Can you work these out from the model? Positions are in its coordinate system, mm. Face numbers are marked on the shaded views. A direction names the side the tool comes from. Give positions to 0.01 mm unless a question says otherwise; leave off trailing zeros. Write each loop counter-clockwise with the first axis right and the second up, starting at its lowest first coordinate (ties: lowest second). Pieces come first, ordered by that corner, then holes. Notation, with made-up numbers: (5.25, 37) -> (42.25, 37) arc R27 cw to (42.25, 64) -> close; hole circle Ø4 at (89, -1). An arc over 180 degrees is marked (long way). One line per item, written item: value.
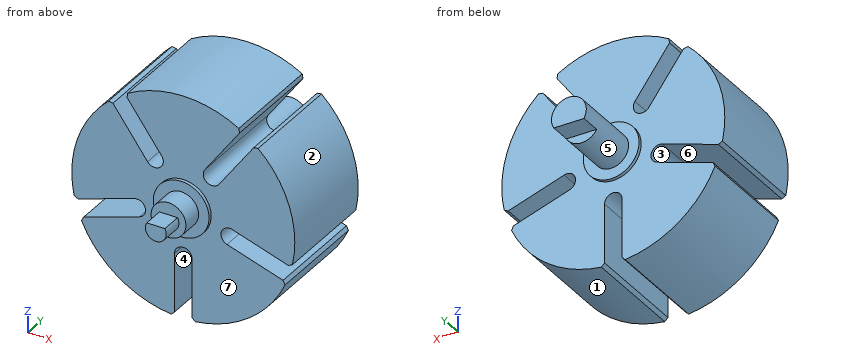
from build123d import *

# Parameters (mm, degrees)
SKETCH_1_R               = 16
EXTRUDE_1_DEPTH          = 15
SKETCH_2_R               = 4
EXTRUDE_2_DEPTH          = 0.5
EXTRUDE_START            = 0.5
SKETCH_3_R               = 4
EXTRUDE_3_DEPTH          = 0.5
SKETCH_4_R               = 2.5
EXTRUDE_4_DEPTH          = 10
EXTRUDE_START_2          = 3
SKETCH_5_R               = 2.5
EXTRUDE_5_DEPTH          = 3
CUT_EXTRUDE_START        = -3
CUT_EXTRUDE_1_DEPTH      = 3
CUT_EXTRUDE_2_DEPTH      = 30.227555491
PATTERN_CIRCULAR_1_COUNT = 5
SKETCH_8_R               = 1.5
EXTRUDE_6_DEPTH          = 3
CHAMFER_1_SIZE           = 0.5
CUT_EXTRUDE_3_DEPTH      = 3


with BuildPart() as part:
    # 草图1 → 凸台-拉伸1 (new body)
    with BuildSketch(Plane(origin=(0, 0, 0), x_dir=(1, 0, 0), z_dir=(0, 1, 0))):
        with Locations(Location((0, 0, 0), (0, 0, 270))):
            Circle(SKETCH_1_R)
    extrude(amount=EXTRUDE_1_DEPTH)

    # 草图2 → 凸台-拉伸2 (add)
    with BuildSketch(Plane(origin=(0, 15, 0), x_dir=(1, 0, 0), z_dir=(0, 1, 0))):
        with Locations(Location((0, 0, 0), (0, 0, 270))):
            Circle(SKETCH_2_R)
    extrude(amount=EXTRUDE_2_DEPTH)

    # 草图3 → 凸台-拉伸3 (add)
    with BuildSketch(Plane.XZ.offset(EXTRUDE_START)):
        with Locations(Location((0, 0, 0), (0, 0, 90))):
            Circle(SKETCH_3_R)
    extrude(amount=-EXTRUDE_3_DEPTH)

    # 草图4 → 凸台-拉伸4 (add)
    with BuildSketch(Plane(origin=(0, 15.5, 0), x_dir=(1, 0, 0), z_dir=(0, 1, 0))):
        with Locations(Location((0, 0, 0), (0, 0, 270))):
            Circle(SKETCH_4_R)
    extrude(amount=EXTRUDE_4_DEPTH)

    # 草图5 → 凸台-拉伸5 (add)
    with BuildSketch(Plane.XZ.offset(0.5).offset(EXTRUDE_START_2)):
        with Locations(Location((0, 0, 0), (0, 0, 90))):
            Circle(SKETCH_5_R)
    extrude(amount=-EXTRUDE_5_DEPTH)

    # 草图6 → 切除-拉伸1 (cut)
    with BuildSketch(Plane(origin=(0, 25.5, 0), x_dir=(1, 0, 0), z_dir=(0, 1, 0)).offset(CUT_EXTRUDE_START)):
        with BuildLine():
            Line((-2.165063509, 1.25), (2.165063509, 1.25))
            ThreePointArc((2.165063509, 1.25), (0, 2.5), (-2.165063509, 1.25))
        make_face()
    extrude(amount=CUT_EXTRUDE_1_DEPTH, mode=Mode.SUBTRACT)

    # 草图7 → 切除-拉伸2 (cut, through all)
    with BuildSketch(Plane(origin=(0, 15, 0), x_dir=(1, 0, 0), z_dir=(0, 1, 0))):
        with BuildLine():
            Line((-1.25, 7), (-1.25, 19))
            Line((-1.25, 19), (1.25, 19))
            Line((1.25, 19), (1.25, 7))
            ThreePointArc((1.25, 7), (0, 5.75), (-1.25, 7))
        make_face()
    cut_extrude_2 = extrude(amount=-CUT_EXTRUDE_2_DEPTH, mode=Mode.SUBTRACT)

    # 阵列(圆周)1: 切除-拉伸2 ×5 about axis
    pattern_circular_1_axis = Axis((0, 0, 0), (0, 1, 0))
    for i in range(1, PATTERN_CIRCULAR_1_COUNT):
        add(cut_extrude_2.rotate(pattern_circular_1_axis, i * 360 / PATTERN_CIRCULAR_1_COUNT), mode=Mode.SUBTRACT)

    # 草图8 → 凸台-拉伸6 (add)
    with BuildSketch(Plane.XZ.offset(3.5)):
        with Locations(Location((0, 0, 0), (0, 0, 270))):
            Circle(SKETCH_8_R)
    extrude(amount=EXTRUDE_6_DEPTH)

    # 倒角1
    # the kernel refuses this chamfer: 0.5, 0.465086612 mm, written as the material it takes off along each edge
    with BuildSketch(Plane(origin=(-1.25, 16.285841494, -15.951097141), x_dir=(-0.9957189737161891, 0, 0.0924322745667282), z_dir=(0, -1, 0)), Plane(origin=(14.784123635, 16.285841494, -6.117980741), x_dir=(-0.3956024015425532, 0, -0.9184218746816544), z_dir=(0, -1, 0)), Plane(origin=(10.3870909, 16.285841494, 12.169977101), x_dir=(0.7512232435318049, 0, -0.6600482091313895), z_dir=(0, -1, 0)), Plane(origin=(-8.364548414, 16.285841494, 13.639440231), x_dir=(0.8598838991841529, 0, 0.5104896472249537), z_dir=(0, -1, 0)), Plane(origin=(-15.556666121, 16.285841494, -3.74033945), x_dir=(-0.21978576745721443, 0, 0.9755481620213546), z_dir=(0, -1, 0))) as chamfer_1_piece_1:
        with BuildLine():
            Line((0.459494947, 0), (CHAMFER_1_SIZE * 0.0924322745667, -CHAMFER_1_SIZE * 0.995718973716))
            Line((CHAMFER_1_SIZE * 0.0924322745667, -CHAMFER_1_SIZE * 0.995718973716), (0, 0))
            ThreePointArc((0, 0), (0.236132262, 0.001648308), (0.459494947, 0))
        make_face()
    extrude(amount=17.571682988, mode=Mode.SUBTRACT)
    with BuildSketch(Plane(origin=(1.25, 16.285841494, -15.951097141), x_dir=(0, 0, 1), z_dir=(0, -1, 0)), Plane(origin=(15.556666121, 16.285841494, -3.74033945), x_dir=(-0.9510565162951534, 0, 0.3090169943749483), z_dir=(0, -1, 0)), Plane(origin=(8.364548414, 16.285841494, 13.639440231), x_dir=(-0.587785252292472, 0, -0.8090169943749483), z_dir=(0, -1, 0)), Plane(origin=(-14.784123635, 16.285841494, -6.117980741), x_dir=(0.9510565162951535, 0, 0.3090169943749477), z_dir=(0, -1, 0))) as chamfer_1_piece_2:
        with BuildLine():
            Line((CHAMFER_1_SIZE, 0), (0.042472163, -0.457527837))
            ThreePointArc((0.042472163, -0.457527837), (0.020184991, -0.235273731), (0, 0))
            Line((0, 0), (CHAMFER_1_SIZE, 0))
        make_face()
    extrude(amount=17.571682988, mode=Mode.SUBTRACT)
    with BuildSketch(Plane(origin=(-10.3870909, 16.285841494, 12.169977101), x_dir=(-0.7512232435318061, 0, -0.6600482091313881), z_dir=(0, -1, 0))) as chamfer_1_piece_3:
        with BuildLine():
            Line((0.459494947, 0), (CHAMFER_1_SIZE * 0.0924322745667, CHAMFER_1_SIZE * 0.995718973716))
            Line((CHAMFER_1_SIZE * 0.0924322745667, CHAMFER_1_SIZE * 0.995718973716), (0, 0))
            ThreePointArc((0, 0), (0.236132262, -0.001648308), (0.459494947, 0))
        make_face()
    extrude(amount=17.571682988, mode=Mode.SUBTRACT)

    # 草图9 → 切除-拉伸3 (cut)
    with BuildSketch(Plane.XZ.offset(6.5).offset(CUT_EXTRUDE_START)):
        with BuildLine():
            Line((-1.299038106, 0.75), (1.299038106, 0.75))
            ThreePointArc((1.299038106, 0.75), (0, 1.5), (-1.299038106, 0.75))
        make_face()
    extrude(amount=CUT_EXTRUDE_3_DEPTH, mode=Mode.SUBTRACT)


solid = part.part
1) If we section it at D-D (y = -4): Write out the boundary of the cut face in (x, z).
Answer list:
outline: (-1.3, 0.75) arc R1.5 ccw (long way) to (1.3, 0.75) -> close
2) Will these pins go through, and if not, where does the flat tip stop? pin 1 (0.8 mm diameter, centred on x = 0.5, y = -4.5, fed in from +Z); pin 2 (2.5 mm diameter, centred on y = 11, z = -10.5, fed in from -X); pin 3 (1 mm diameter, centred on x = 5, y = 1.5, fed in from +Z).
Answer list:
pin 1: stops at z = 0.75
pin 2: stops at x = -13.06
pin 3: stops at z = 15.35
3) I need wall thicknesses on L1, parallel to Z at x = -6, y = 12.5; L2, parallel to X at y = 3, z = 5; L3, parallel to Y at x = -1.5, z = -11. Which ranges of each line are inside material? Lowest first, please.
Answer list:
L1: z = -14.83 to -3.23, -1.1 to 6.13, 10.38 to 14.83
L2: x = -15.2 to -5.18, -3.05 to 3.05, 5.18 to 15.2
L3: y = 0 to 15
4) We'd pull the mould along Z, two halves only. Please class the marked faces 1, 2 and 3: released by +Z, released by -Z, zero draft, split by the parting line, or undercut.
Answer list:
face 1: released by -Z
face 2: split by the parting line
face 3: undercut
5) For the marked faces 4, 5, 6 and 7, which set-ups out of +Z, -Z, +X, -X, +Y, -Y let a thin tool reach every point of the face, with its end or its side?
Answer list:
face 4: -Z, +Y, -Y
face 5: +Y
face 6: +Y, -Y
face 7: -Y
6) If we section it at C-C (z = 0): Write out the boundary of the cut face in (x, y).
Answer list:
outline: (-16, 0) -> (-4, 0) -> (-4, -0.5) -> (-2.5, -0.5) -> (-2.5, -3.5) -> (-1.5, -3.5) -> (-1.5, -6.5) -> (1.5, -6.5) -> (1.5, -3.5) -> (2.5, -3.5) -> (2.5, -0.5) -> (4, -0.5) -> (4, 0) -> (16, 0) -> (16, 15) -> (4, 15) -> (4, 15.5) -> (2.5, 15.5) -> (2.5, 25.5) -> (-2.5, 25.5) -> (-2.5, 15.5) -> (-4, 15.5) -> (-4, 15) -> (-16, 15) -> close
7) If we section it at A-A (z = 9.5): Write out the boundary of the cut face in (x, y), and give its area (3 significant figures).
Answer list:
outline: (-12.87, 0) -> (-8.45, 0) -> (-8.45, 15) -> (-12.87, 15) -> close; (-5.36, 0) -> (5.36, 0) -> (5.36, 15) -> (-5.36, 15) -> close; (8.45, 0) -> (12.87, 0) -> (12.87, 15) -> (8.45, 15) -> close
area: 294 mm^2
